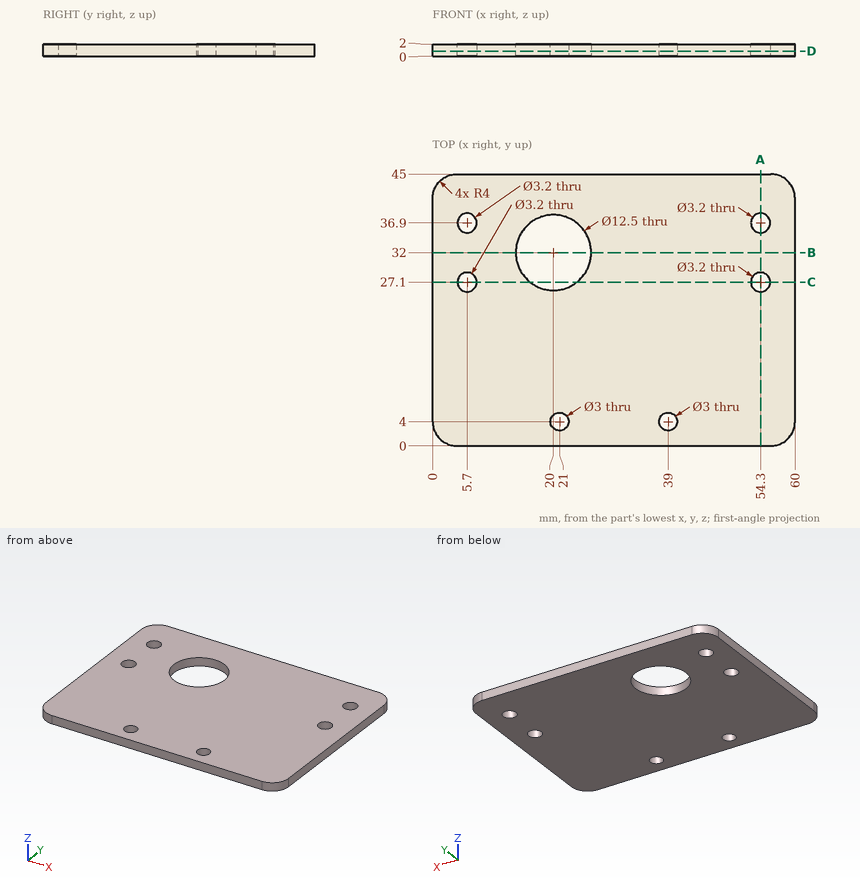
The figure shows three views and two pictorial views of one solid part (mm, origin at its lowest corner). Answer the questions. Give positions to 0.01 mm unless a question says otherwise; leave off trailing zeros. Write each loop counter-clockwise with the first axis right and the second up, starting at its lowest first coordinate (ties: lowest second). Pieces come first, ordered by that corner, then holes.
Q1. The part is cut by section D-D on z = 0.8. Give the vertices of the cut face in (x, y).
Answer:
outline: (0, 4) arc R4 ccw to (4, 0) - (56, 0) arc R4 ccw to (60, 4) - (60, 41) arc R4 ccw to (56, 45) - (4, 45) arc R4 ccw to (0, 41) - close; hole circle Ø3.2 at (5.7, 27.1); hole circle Ø3.2 at (5.7, 36.9); hole circle Ø12.5 at (20, 32); hole circle Ø3 at (21, 4); hole circle Ø3 at (39, 4); hole circle Ø3.2 at (54.3, 27.1); hole circle Ø3.2 at (54.3, 36.9)
Q2. Given pin 1 (3.5 mm diameter, centred on x = 21, y = 4, fed in from +Z), flat-ended and moving along its own axis, determine where the tip first touches the part or whether it passes through.
Answer:
pin 1: stops at z = 2
Q3. The part is cut by section B-B on y = 32. Give the vertices of the cut face in (x, z), and give its area (3 significant figures).
Answer:
outline: (0, 0) - (13.75, 0) - (13.75, 2) - (0, 2) - close; (26.25, 0) - (60, 0) - (60, 2) - (26.25, 2) - close
area: 95.0 mm2
Q4. Straight lines are drawn through the part: L1, parallel to Y at x = 54.3, z = 0.6; L2, parallel to Y at x = 21, z = 1; L3, parallel to Y at x = 39, z = 1.55. For each, find the intervals that lie inside material, in ascending order.
Answer:
L1: y = 0 to 25.5, 28.7 to 35.3, 38.5 to 45
L2: y = 0 to 2.5, 5.5 to 25.83, 38.17 to 45
L3: y = 0 to 2.5, 5.5 to 45
Q5. The part is cut by section A-A on x = 54.3. Give the vertices of the cut face in (y, z), and give its area (3 significant figures).
Answer:
outline: (0, 0) - (25.5, 0) - (25.5, 2) - (0, 2) - close; (28.7, 0) - (35.3, 0) - (35.3, 2) - (28.7, 2) - close; (38.5, 0) - (45, 0) - (45, 2) - (38.5, 2) - close
area: 77.2 mm2
Q6. The part is cut by section C-C on y = 27.1. Give the vertices of the cut face in (x, z), and give its area (3 significant figures).
Answer:
outline: (0, 0) - (4.1, 0) - (4.1, 2) - (0, 2) - close; (7.3, 0) - (16.12, 0) - (16.12, 2) - (7.3, 2) - close; (23.88, 0) - (52.7, 0) - (52.7, 2) - (23.88, 2) - close; (55.9, 0) - (60, 0) - (60, 2) - (55.9, 2) - close
area: 91.7 mm2
